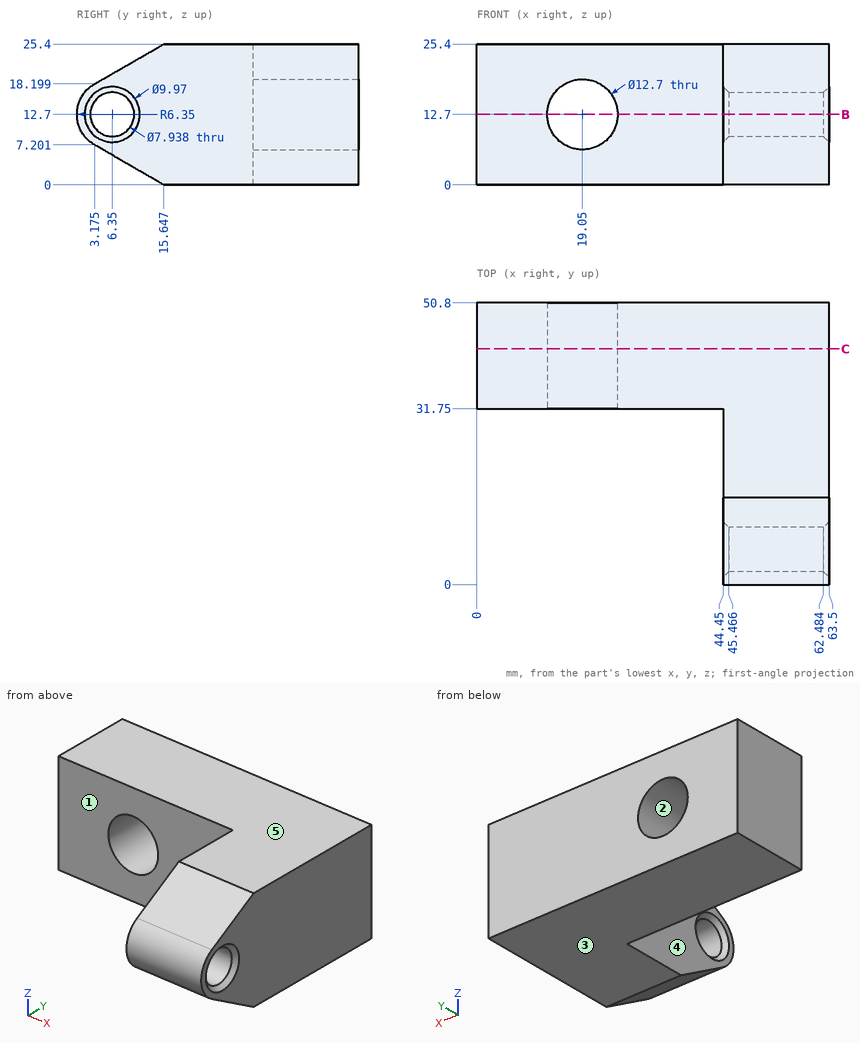
The figure shows three views and two pictorial views of one solid part (mm, origin at its lowest corner). Answer the questions. A direction names the side the tool comes from. Give positions to 0.01 mm unless a question says otherwise; leave off trailing zeros. Loops run counter-clockwise (first coordinate to the right, second up) from the corner with the lowest first, then second, coordinate; pieces in that order, holes last. Notation, with made-up numbers: (30, 39) -> (57, 39) arc R22 ccw to (57, 68) -> close; hole circle Ø2 at (86, 87). An arc over 180 degrees is marked (long way). Use a Markdown table: item, result. Add a question column.
1. Section C-C on y = 42.5 is taken. Determine the outline of the cut face in (x, z), and give its area (3 significant figures).
2. Find the intervals of material crossed by probe 1 along Z at (x, y) = (19, 46); probe 2 along Y at (x, z) = (6.5, 9.5); probe 3 along Z at (x, y) = (17.5, 46.5), in increasing order.
3. Section B-B on z = 12.7 is taken. State how many separate pieces and enclosed holes the cut face has, and give its area (3 significant figures).
4. For the marked faces 4 and 5, determine the directions among +Z, -Z, +X, -X, +Y, -Y from which every point of the face is accessible in a straight line to the end or side of a thin tool.
5. Flat-ended cylindrical pins translate along their axes: pin 1 Ø4 at (x, z) = (37, 6) entering from -Y; pin 2 Ø10 at (x, y) = (53.5, 29) entering from -Z; pin 3 Ø5 at (y, z) = (16, 21) entering from -X. Find the tip coordinate at first contact, or state that the pin passes through.
6. Determine the mould class of the marked faces 1, 2 and 3 for opening direction Z: released by +Z, released by -Z, zero draft, split by the parting line, or undercut.
Results below:
| question | item | result |
|---|---|---|
| 1 | outline | (0, 0) -> (63.5, 0) -> (63.5, 25.4) -> (0, 25.4) -> close; hole circle Ø12.7 at (19.05, 12.7) |
| 1 | area | 1,490 mm^2 |
| 2 | probe 1 | z = 0 to 6.35, 19.05 to 25.4 |
| 2 | probe 2 | y = 31.75 to 50.8 |
| 2 | probe 3 | z = 0 to 6.54, 18.86 to 25.4 |
| 3 | separate pieces | 3 |
| 3 | enclosed holes | 0 |
| 3 | area | 1,420 mm^2 |
| 4 | face 4 | +Z, -Z, -X, -Y |
| 4 | face 5 | +Z, +X, -X, +Y, -Y |
| 5 | pin 1 | stops at y = 31.75 |
| 5 | pin 2 | stops at z = 0 |
| 5 | pin 3 | stops at x = 44.45 |
| 6 | face 1 | zero draft |
| 6 | face 2 | undercut |
| 6 | face 3 | released by -Z |
